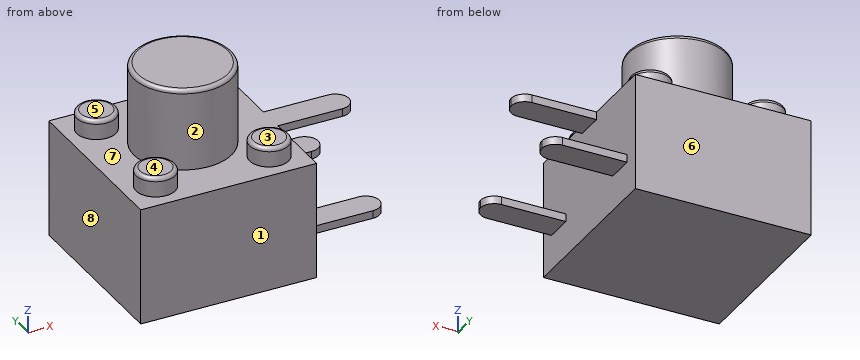
```python
from build123d import *

# Parameters (mm, degrees)
SKETCH1_W           = 4.5
SKETCH1_H           = 4.5
BOSS_EXTRUDE1_DEPTH = 3
SKETCH4_R           = 0.5
BOSS_EXTRUDE3_DEPTH = 0.5
FILLET1_R           = 0.1
SKETCH5_R           = 1.25
BOSS_EXTRUDE4_DEPTH = 2.1
FILLET2_R           = 0.1
SKETCH6_W           = 2
SKETCH6_H           = 0.7
BOSS_EXTRUDE5_DEPTH = 0.2
SKETCH7_W           = 2
SKETCH7_H           = 0.7
BOSS_EXTRUDE6_DEPTH = 0.1
FILLET3_R           = 0.35


with BuildPart() as part:
    # Sketch1 → Boss-Extrude1 (new body)
    with BuildSketch(Plane.XY):
        Rectangle(SKETCH1_W, SKETCH1_H)
    extrude(amount=BOSS_EXTRUDE1_DEPTH)

    # Sketch4 → Boss-Extrude3 (add)
    with BuildSketch(Plane.XY.offset(3)):
        with Locations(Location((-1.45218189, 1.45218189, 0), (0, 0, 180))):
            Circle(SKETCH4_R)
        with Locations(Location((1.45218189, 1.45218189, 0), (0, 0, 180))):
            Circle(SKETCH4_R)
        with Locations(Location((1.45218189, -1.45218189, 0), (0, 0, 180))):
            Circle(SKETCH4_R)
        with Locations(Location((-1.45218189, -1.45218189, 0), (0, 0, 180))):
            Circle(SKETCH4_R)
    extrude(amount=BOSS_EXTRUDE3_DEPTH)

    # Fillet1
    fillet1_edges = [part.edges().sort_by_distance(p)[0] for p in [
        (-0.95218189, 1.45218189, 3.5),
        (1.95218189, 1.45218189, 3.5),
        (1.95218189, -1.45218189, 3.5),
        (-0.95218189, -1.45218189, 3.5),
    ]]
    fillet(fillet1_edges, radius=FILLET1_R)

    # Sketch5 → Boss-Extrude4 (add)
    with BuildSketch(Plane.XY.offset(3)):
        with Locations(Location((0, 0, 0), (0, 0, 180))):
            Circle(SKETCH5_R)
    extrude(amount=BOSS_EXTRUDE4_DEPTH)

    # Fillet2
    fillet2_edges = [part.edges().sort_by_distance(p)[0] for p in [
        (1.25, 0, 5.1),
    ]]
    fillet(fillet2_edges, radius=FILLET2_R)

    # Sketch6 → Boss-Extrude5 (add)
    with BuildSketch(Plane.XY.offset(3)):
        with Locations((3.25, 0)):
            Rectangle(SKETCH6_W, SKETCH6_H)
    extrude(amount=-BOSS_EXTRUDE5_DEPTH)

    # Sketch7 → Boss-Extrude6 (add, symmetric)
    with BuildSketch(Plane(origin=(0, 0, 1), x_dir=(-1, 0, 0), z_dir=(0, 0, -1))):
        with Locations((-3.25, -1.5)):
            Rectangle(SKETCH7_W, SKETCH7_H)
        with Locations((-3.25, 1.5)):
            Rectangle(SKETCH7_W, SKETCH7_H)
    extrude(amount=BOSS_EXTRUDE6_DEPTH, both=True)

    # Fillet3
    fillet3_edges = [part.edges().sort_by_distance(p)[0] for p in [
        (4.25, 1.85, 1),
        (4.25, 1.15, 1),
        (4.25, -0.35, 2.9),
        (4.25, 0.35, 2.9),
        (4.25, -1.15, 1),
        (4.25, -1.85, 1),
    ]]
    fillet(fillet3_edges, radius=FILLET3_R - 0.0001)  # a hair under: the kernel refuses the full size


solid = part.part
```
CAD build for the part. Positions are in the model's coordinates, mm. Face numbers are marked on the shaded views. A direction names the side the tool comes from. Round coordinates to 2 decimals unless told otherwise and drop trailing zeros. Loops run counter-clockwise (first coordinate to the right, second up) from the corner with the lowest first, then second, coordinate; pieces in that order, holes last. Notation, with made-up numbers: (-16.75, 16) - (37.25, 16) arc R32 ccw to (37.25, 42) - close; hole circle Ø7 at (14, 10.25). An arc over 180 degrees is marked (long way). Return JSON: item names as keys, results as strings. Group by question number.
Q1. Band-saw the part on A-A on x = 3.25. Give the cut face in (y, z).
Q2. Band-saw the part on C-C on z = 3.2. Give the cut face in (x, y), plus the area to 3 significant figures.
Q3. Tool access for the marked faces 1, 2, 3, 4 and 5: list every direction of +Z, -Z, +X, -X, +Y, -Y with a clear straight run to the whole face (end or side of a thin tool).
Q4. Band-saw the part on D-D on x = 4. Give the cut face in (y, z).
Q5. Band-saw the part on B-B on x = 0. Give the cut face in (y, z).
Q6. Flat gauge pins, fed straight in: pin 1 Ø0.6 at (x, y) = (3.5, 0) entering from -Z; pin 2 Ø0.6 at (x, y) = (1.5, 1.5) entering from +Z; pin 3 Ø0.6 at (x, y) = (3.5, -1.5) entering from -Z. Where does each tip first touch, or does it go through?
Q7. Two-plate mould, pull along X, no slides. Class the marked faces 6, 7 and 8: +X half, -X half, draft (parallel to the pull), parting line (faces both ways), or undercut.
Q8. Drill centre lines: line 1 along Z through (x, y) = (2, -0.45); line 2 along X through (y, z) = (0.05, 4); line 3 along X through (y, z) = (-0.2, 0.4). Where is each one in solid material? Low to high. Write a range as [from, to].
Solutions:
{
 "1": {"outline": "(-1.85, 0.9) - (-1.15, 0.9) - (-1.15, 1.1) - (-1.85, 1.1) - close; (-0.35, 2.8) - (0.35, 2.8) - (0.35, 3) - (-0.35, 3) - close; (1.15, 0.9) - (1.85, 0.9) - (1.85, 1.1) - (1.15, 1.1) - close"},
 "2": {"outline": "circle Ø1 at (-1.45, -1.45); circle Ø1 at (-1.45, 1.45); circle Ø2.5 at (0, 0); circle Ø1 at (1.45, -1.45); circle Ø1 at (1.45, 1.45)", "area": "8.05 mm^2"},
 "3": {"face 1": "+Z, -Z, +X, -X, -Y", "face 2": "+Z", "face 3": "+Z, +X, -Y", "face 4": "+Z, -X, -Y", "face 5": "+Z, -X, +Y"},
 "4": {"outline": "(-1.84, 0.9) - (-1.16, 0.9) - (-1.16, 1.1) - (-1.84, 1.1) - close; (-0.34, 2.8) - (0.34, 2.8) - (0.34, 3) - (-0.34, 3) - close; (1.16, 0.9) - (1.84, 0.9) - (1.84, 1.1) - (1.16, 1.1) - close"},
 "5": {"outline": "(-2.25, 0) - (2.25, 0) - (2.25, 3) - (1.25, 3) - (1.25, 5) arc R0.1 ccw to (1.15, 5.1) - (-1.15, 5.1) arc R0.1 ccw to (-1.25, 5) - (-1.25, 3) - (-2.25, 3) - close"},
 "6": {"pin 1": "stops at z = 2.8", "pin 2": "stops at z = 3.5", "pin 3": "stops at z = 0.9"},
 "7": {"face 6": "draft", "face 7": "undercut", "face 8": "-X half"},
 "8": {"line 1": "z = [0, 3]", "line 2": "x = [-1.25, 1.25]", "line 3": "x = [-2.25, 2.25]"}
}
